Read the model definition and answer for the solid it produces. Units are mm, in the model's axes. Give positions to 0.01 mm unless a question says otherwise; leave off trailing zeros. Write each loop counter-clockwise with the first axis right and the second up, starting at its lowest first coordinate (ties: lowest second). Pieces come first, ordered by that corner, then holes. Notation, with made-up numbers: M -36.5,-11 L -29.5,-11 A20 ccw -29.5,23 Z; hole C 25.25,62.25 d9. An arc over 180 degrees is marked long. Answer as CSV lines item,"result". Start each with the question number.
```python
from build123d import *

# Parameters (mm, degrees)
F0_W     = 120
F0_H     = 132
F0_R     = 1.9
F0_R_2   = 4
F0_H_2   = 50
F0_R_3   = 1.55
F0_R_4   = 6.5
F1_DEPTH = 5
F2_R     = 4
F3_DEPTH = 25


# Not quite as in the source:
# - a feature names something its author has since deleted; it is built from what else it names


with BuildPart() as f1:
    # F0 (on Top) → F1 (new body)
    with BuildSketch(Plane.XY):
        Rectangle(F0_W, F0_H)
        with Locations((-52, -50)):
            Circle(F0_R, mode=Mode.SUBTRACT)
        with Locations((-20, -50)):
            Circle(F0_R, mode=Mode.SUBTRACT)
        with Locations((-3, -50)):
            Circle(F0_R_2, mode=Mode.SUBTRACT)
        with Locations((12, -50)):
            Circle(F0_R, mode=Mode.SUBTRACT)
        with Locations((44, -50)):
            Circle(F0_R, mode=Mode.SUBTRACT)
        with Locations((0, 91)):
            Rectangle(F0_W, F0_H_2)
        with Locations((-15.5, 91)):
            Circle(F0_R_3, mode=Mode.SUBTRACT)
        with Locations((-7.75, 77.5766062413)):
            Circle(F0_R_3, mode=Mode.SUBTRACT)
        with Locations((-7.75, 104.4233937587)):
            Circle(F0_R_3, mode=Mode.SUBTRACT)
        with Locations((7.75, 77.5766062413)):
            Circle(F0_R_3, mode=Mode.SUBTRACT)
        with Locations((6.9857463241, 91)):
            Circle(F0_R_4, mode=Mode.SUBTRACT)
        with Locations((15.5, 91)):
            Circle(F0_R_3, mode=Mode.SUBTRACT)
        with Locations((7.75, 104.4233937587)):
            Circle(F0_R_3, mode=Mode.SUBTRACT)
    extrude(amount=F1_DEPTH)

    # F2 (on face) → F3 (cut)
    with BuildSketch(Plane.XY.offset(5)):
        with Locations((0, 21)):
            Circle(F2_R)
    extrude(amount=-F3_DEPTH, mode=Mode.SUBTRACT)


solid = f1.part
```
1. Find section A-A on x = 44. Determine the outline of the cut face in (y, z).
2. Find the intervals of material crossed by line 1 (Y direction, x = 12, z = 1.65); line 2 (Y direction, x = 15.5, z = 3.3); line 3 (X direction, y = -49.5, z = 3.4), in increasing order. Write a range as [from, to].
3. Find section B-B on y = -50. Determine the outline of the cut face in (x, z), then the cut area to 3 significant figures.
4. Given pin 1 (3 mm diameter, centred on x = 15.5, y = 29, fed in from -Z), flat-ended and moving along its own axis, determine where the tip first touches the part or whether it passes through.
5. Determine the mould class of faces 1 (the face through (60, 24, 2)), 2 (the face through (5.577, 84.655, 2.465)), 3 (the face through (-1, -66, 2)), 4 (the face through (-20.412, -51.855, 2.465)) for opening direction X: +X half, -X half, draft (parallel to the pull), parting line (faces both ways), or undercut.
6. Find section C-C on x = -1.5. Determine the outline of the cut face in (y, z), then the cut area to 3 significant figures.
Computed:
1,outline,"M -66,0 L -51.9,0 L -51.9,5 L -66,5 Z; M -48.1,0 L 116,0 L 116,5 L -48.1,5 Z"
2,line 1,"y = [-66, -51.9], [-48.1, 86.86], [95.14, 116]"
2,line 2,"y = [-66, 89.45], [92.55, 116]"
2,line 3,"x = [-60, -53.83], [-50.17, -21.83], [-18.17, -6.97], [0.97, 10.17], [13.83, 42.17], [45.83, 60]"
3,outline,"M -60,0 L -53.9,0 L -53.9,5 L -60,5 Z; M -50.1,0 L -21.9,0 L -21.9,5 L -50.1,5 Z; M -18.1,0 L -7,0 L -7,5 L -18.1,5 Z; M 1,0 L 10.1,0 L 10.1,5 L 1,5 Z; M 13.9,0 L 42.1,0 L 42.1,5 L 13.9,5 Z; M 45.9,0 L 60,0 L 60,5 L 45.9,5 Z"
3,area,"484 mm^2"
4,pin 1,"stops at z = 0"
5,face 1,"+X half"
5,face 2,"undercut"
5,face 3,"draft"
5,face 4,"undercut"
6,outline,"M -66,0 L -53.71,0 L -53.71,5 L -66,5 Z; M -46.29,0 L 17.29,0 L 17.29,5 L -46.29,5 Z; M 24.71,0 L 116,0 L 116,5 L 24.71,5 Z"
6,area,"836 mm^2"
